```python
from build123d import *

# Parameters (mm, degrees)
F0_R     = 29.6029222689
F1_DEPTH = 12.7
F2_R     = 5.08
F3_DEPTH = 25.4


with BuildPart() as f1:
    # F0 (on Top) → F1 (new body, symmetric)
    with BuildSketch(Plane.XY):
        Circle(F0_R)
    extrude(amount=F1_DEPTH, both=True)

    # F2
    f2_edges = [f1.edges().sort_by_distance(p)[0] for p in [
        (-29.602922, 0, 12.7),
        (-29.602922, 0, -12.7),
    ]]
    fillet(f2_edges, radius=F2_R)

    # F3 (add): a face of the model
    f3_faces = [f1.faces().sort_by_distance(p)[0] for p in [
        (0, 0, 12.7),
    ]]
    extrude(f3_faces, amount=F3_DEPTH)


solid = f1.part
```
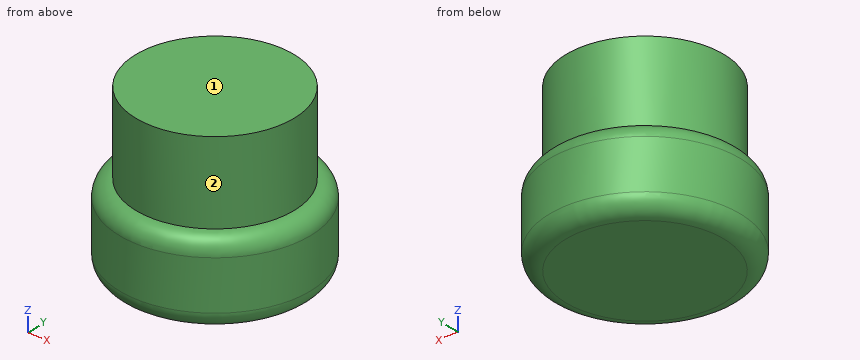
Here's how the part is built. I have some questions about the finished solid (model axes, mm). Face numbers are marked on the shaded views. Coordinates: 2 decimals unless noted, no trailing zeros. Order: outer loops, then holes, each group sorted by start corner. A loop starts at its lowest first (then second) coordinate and runs counter-clockwise, first axis right, second up.
1) We'd pull the mould along X, two halves only. Please class the marked faces 1 and 2: +X half, -X half, draft (parallel to the pull), parting line (faces both ways), or undercut.
2) Imagine slicing it at A-A on y = 0. List the corners of the cut face in (x, z) for me.
3) Imagine slicing it at D-D on z = -3. List the corners of the cut face in (x, y) for me.
4) I need wall thicknesses on line 1 (X direction, y = 9, z = 3.5); line 2 (X direction, y = -4, z = -10); line 3 (Y direction, x = -22, z = 13.5). Which ranges of each line are inside material? Lowest first, please.
5) Will these pins go through, and if not, where does the flat tip stop? pin 1 (3 mm diameter, centred on x = -21, z = 13, fed in from +Y); pin 2 (3 mm diameter, centred on y = -19.5, z = 6, fed in from -X); pin 3 (10 mm diameter, centred on x = 18.5, z = 8.5, fed in from +Y).
6) Imagine slicing it at C-C on z = 24. List the corners of the cut face in (x, y) for me.
Response values:
1. face 1: draft
1. face 2: parting line
2. outline: (-29.6, -7.62) arc R5.08 ccw to (-24.52, -12.7) - (24.52, -12.7) arc R5.08 ccw to (29.6, -7.62) - (29.6, 7.62) arc R5.08 ccw to (24.52, 12.7) - (24.52, 38.1) - (-24.52, 38.1) - (-24.52, 12.7) arc R5.08 ccw to (-29.6, 7.62) - close
3. outline: circle Ø59.21 at (0, 0)
4. line 1: x = -28.2 to 28.2
4. line 2: x = -28.73 to 28.73
4. line 3: y = -10.83 to 10.83
5. pin 1: stops at y = 18.68
5. pin 2: stops at x = -23.5
5. pin 3: stops at y = 26.32
6. outline: circle Ø49.05 at (0, 0)
